Verification items for the finished model (mm, model axes). Face numbers are marked on the shaded views. A direction names the side the tool comes from. Coordinates: 2 decimals unless noted, no trailing zeros. Order: outer loops, then holes, each group sorted by start corner. A loop starts at its lowest first (then second) coordinate and runs counter-clockwise, first axis right, second up. Notation, with made-up numbers: M 13,84 L 22,84 A27 cw 22,108 Z; hole C 60,39.5 d4. An arc over 180 degrees is marked long. Return JSON: item names as keys, results as strings.
```python
from build123d import *

# Parameters (mm, degrees)
BOSS_EXTRUDE1_DEPTH = 1.905
SKETCH2_R           = 3.048
BOSS_EXTRUDE2_DEPTH = 14.9098


with BuildPart() as part:
    # Sketch1 → Boss-Extrude1 (new body)
    with BuildSketch(Plane(origin=(0, 0, 0), x_dir=(1, 0, 0), z_dir=(0, 1, 0))):
        Polygon((-6.096, 9.017), (6.096, 9.017), (9.017, 6.096), (9.017, -6.096), (6.096, -9.017), (-6.096, -9.017), (-9.017, -6.096), (-9.017, 6.096), align=None)
    extrude(amount=BOSS_EXTRUDE1_DEPTH)

    # Sketch2 → Boss-Extrude2 (add)
    with BuildSketch(Plane(origin=(0, 1.905, 0), x_dir=(1, 0, 0), z_dir=(0, 1, 0))):
        Circle(SKETCH2_R)
    extrude(amount=BOSS_EXTRUDE2_DEPTH)


solid = part.part
```
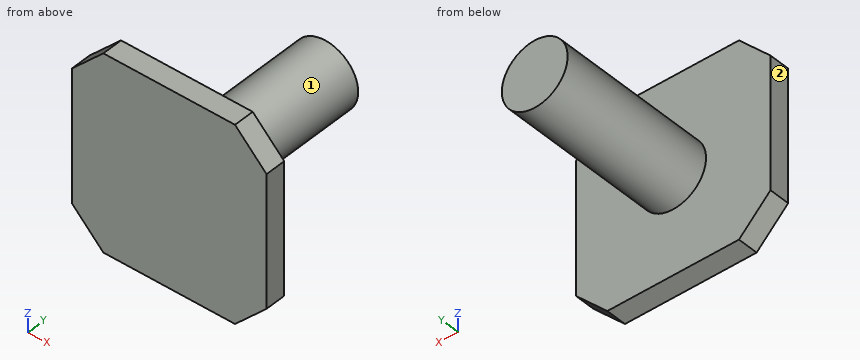
Q1. Cross-section at D-D, the plane x = -5.75. Record the boundary of the cut face in (y, z) (3 decimals).
Values:
{"outline": "M 0,-9.017 L 1.905,-9.017 L 1.905,9.017 L 0,9.017 Z"}
Q2. Cross-section at B-B, the plane x = 0. Record the boundary of the cut face in (y, z) (3 decimals).
Values:
{"outline": "M 0,-9.017 L 1.905,-9.017 L 1.905,-3.048 L 16.815,-3.048 L 16.815,3.048 L 1.905,3.048 L 1.905,9.017 L 0,9.017 Z"}
Q3. Cross-section at A-A, the plane z = 0. Record the boundary of the cut face in (x, y) (3 decimals).
Values:
{"outline": "M -9.017,0 L 9.017,0 L 9.017,1.905 L 3.048,1.905 L 3.048,16.815 L -3.048,16.815 L -3.048,1.905 L -9.017,1.905 Z"}
Q4. Tool access check on the marked faces 1 and 2. Record the directions out of +Z, -Z, +X, -X, +Y, -Y that give a thin tool (end or side, any length) a straight path to the whole face; none if there is none.
Values:
{"face 1": "+Y", "face 2": "+Z, -Z, -X, +Y, -Y"}
Q5. Go/stop test with flat-tipped pins: pin 1 (1.5 mm diameter, centred on x = -3, z = 4, fed in from -Y); pin 2 (1 mm diameter, centred on y = 6.5, z = 0.5, fed in from +X); pin 3 (5 mm diameter, centred on x = 5, y = 9, fed in from +Z); pin 4 (3 mm diameter, centred on x = 3.5, y = 8, fed in from +Z). Record where each tip stops, or that it passes through.
Values:
{"pin 1": "y = 0", "pin 2": "x = 3.05", "pin 3": "z = 1.74", "pin 4": "z = 2.3"}
Q6. Material ranges on line 1 along Y through (x, z) = (6.75, -4.25) (3 decimals); line 2 along X through (y, z) = (1, 7.5); line 3 along Z through (x, y) = (1.5, 9.25), recorded low to high.
Values:
{"line 1": "0 to 1.905", "line 2": "-7.61 to 7.61", "line 3": "-2.65 to 2.65"}
Q7. Cross-section at C-C, the plane y = 3.5. Record the boundary of the cut face in (x, z).
Values:
{"outline": "C 0,0 d6.1"}
